For this review, take the finished solid that the model builds, in its own axes (mm). A direction names the side the tool comes from. Coordinates: 2 decimals unless noted, no trailing zeros. Order: outer loops, then holes, each group sorted by start corner. A loop starts at its lowest first (then second) coordinate and runs counter-clockwise, first axis right, second up. Notation, with made-up numbers: M 37,60.5 L 91,60.5 A17 ccw 91,81.5 Z; hole C 58.25,8.5 d4. An arc over 180 degrees is marked long. Use CSV: the item, a comma, the result in double quotes.
Autodesk Inventor part; units mm, degrees
ref_plane "YZ Plane" through (0, 0, 0) normal (1, 0, 0) x (0, 1, 0)
ref_plane "XZ Plane" through (0, 0, 0) normal (0, 1, 0) x (-1, 0, 0)
ref_plane "XY Plane" through (0, 0, 0) normal (0, 0, 1) x (1, 0, 0)
sketch "Sketch1" plane through (0, 0, 0) normal (0, 0, 1) x (1, 0, 0)
  line L0 (0, -3) -> (0, -30)
  line L1 (0, -30) -> (-3, -30)
  line L2 (-3, 0) -> (-30, 0)
  line L3 (-30, 0) -> (-30, -3)
  line L4 (-30, -3) -> (-5, -3)
  line L5 (-3, -5) -> (-3, -30)
  arc A0 (-3, -5) -> (-5, -3) centre (-5, -5) ccw
  arc A1 (0, -3) -> (-3, 0) centre (-3, -3) ccw
  point P0 (0, 0)
  dimension "d0" = 3
  dimension "d1" = 30
  dimension "d2" = 30
  dimension "d3" = 3
  dimension "d4" = 2
  dimension "d5" = 3
extrude "Extrusion1" add sketch "Sketch1" along normal blind 10
sketch "Sketch2" plane through (-30, 0, 0) normal (0, 1, 0) x (1, 0, 0)
  line L0 (0, 0) -> (0, -10)
  line L1 (0, -5) -> (105.7615, -5) construction
  circle A0 centre (6, -5) radius 1.5
  circle A1 centre (21, -5) radius 1.5
  point P0 (30, 0)
  dimension "d8" = 3
  dimension "d9" = 3
  dimension "d10" = 6
  dimension "d11" = 15
extrude "Extrusion2" cut sketch "Sketch2" against normal blind 3
equation "\"d3\" = d0"
equation "\"d9\" = d8"
properties part number "profiletto a l"
Item 1: Add section B-B on z = 5. State the section outline as (x, y) points.
Solutions:
outline,"M -30,-3 L -25.5,-3 L -25.5,0 L -30,0 Z; M -22.5,-3 L -10.5,-3 L -10.5,0 L -22.5,0 Z; M -7.5,-3 L -5,-3 A2 cw -3,-5 L -3,-30 L 0,-30 L 0,-3 A3 ccw -3,0 L -7.5,0 Z"
Item 2: Add section D-D on x = -10. State the section outline as (y, z) points.
Solutions:
outline,"M -3,0 L 0,0 L 0,3.88 L -3,3.88 Z; M -3,6.12 L 0,6.12 L 0,10 L -3,10 Z"
Item 3: Add section A-A on x = -24. State the section outline as (y, z) points, and give its area (3 significant figures).
Solutions:
outline,"M -3,0 L 0,0 L 0,3.5 L -3,3.5 Z; M -3,6.5 L 0,6.5 L 0,10 L -3,10 Z"
area,"21.0 mm^2"
Item 4: For faces 1 (the face through (-18, -3, 5)), 2 (the face through (-30, -1, 5)), list the 3-axis set-ups (+Z, -Z, +X, -X, +Y, -Y) from which the entire face can be reached by the end or side of a thin tool; tool diameter is ignored.
Solutions:
face 1,"+Z, -Z, -X, -Y"
face 2,"+Z, -Z, -X, +Y, -Y"
Item 5: Add section C-C on z = 7. State the section outline as (x, y) points, and give its area (3 significant figures).
Solutions:
outline,"M -30,-3 L -5,-3 A2 cw -3,-5 L -3,-30 L 0,-30 L 0,-3 A3 ccw -3,0 L -30,0 Z"
area,"170 mm^2"
Item 6: Clearance check with flat-ended pins moving along their axes: pin 1 Ø3 at (y, z) = (-22, 3) entering from -X; pin 2 Ø5 at (x, z) = (-9, 5) entering from -Y. State where each tip first meets the part, or that it passes through.
Solutions:
pin 1,"x = -3"
pin 2,"y = -3"
Item 7: Draft analysis for pull direction X (two halves, no side actions). For faces 3 (the face through (-10.5, -1.48, 4.93)), 4 (the face through (-25.5, -1.48, 4.93)), 5 (the face through (-0.9, -0.86, 4.93)), 6 (the face through (-3, -17, 5)), state which applies: released by +X, released by -X, zero draft, split by the parting line, or undercut.
Solutions:
face 3,"undercut"
face 4,"undercut"
face 5,"released by +X"
face 6,"released by -X"
Item 8: To check wall thickness, follow line 1 along Z through (x, y) = (-9, -1.05); line 2 along X through (y, z) = (-1.4, 5); line 3 along X through (y, z) = (-1.15, 5). State the ranges of each line that lie inside material, in increasing order. Write a range as [from, to].
Solutions:
line 1,"[0, 3.5], [6.5, 10]"
line 2,"[-30, -25.5], [-22.5, -10.5], [-7.5, -0.46]"
line 3,"[-30, -25.5], [-22.5, -10.5], [-7.5, -0.64]"
